Design review of the part built by this model. Coordinates are the model's own, in mm. A direction names the side the tool comes from. Give positions to 0.01 mm unless a question says otherwise; leave off trailing zeros. Write each loop counter-clockwise with the first axis right and the second up, starting at its lowest first coordinate (ties: lowest second). Pieces come first, ordered by that corner, then holes. Notation, with made-up numbers: (2, 74.5) -> (36, 74.5) arc R5 ccw to (36, 78.5) -> close; hole circle Ø8 at (37.5, 26.25). An arc over 180 degrees is marked (long way). Use CSV: the item, a comma, the result in double quotes.
```python
from build123d import *

# Parameters (mm, degrees)
SKETCH1_R           = 2.725
BOSS_EXTRUDE1_DEPTH = 2.9
SKETCH2_R           = 1.475
BOSS_EXTRUDE2_DEPTH = 10
CUT_EXTRUDE1_DEPTH  = 1.75


with BuildPart() as part:
    # Sketch1 → Boss-Extrude1 (new body)
    with BuildSketch(Plane(origin=(0, 0, 0), x_dir=(1, 0, 0), z_dir=(0, 1, 0))):
        Circle(SKETCH1_R)
    extrude(amount=BOSS_EXTRUDE1_DEPTH)

    # Sketch2 → Boss-Extrude2 (add)
    with BuildSketch(Plane.XZ):
        Circle(SKETCH2_R)
    extrude(amount=BOSS_EXTRUDE2_DEPTH)

    # Sketch3 → Cut-Extrude1 (cut)
    with BuildSketch(Plane(origin=(0, 2.9, 0), x_dir=(1, 0, 0), z_dir=(0, 1, 0))):
        Polygon((0, 1.443375673), (-1.25, 0.721687836), (-1.25, -0.721687836), (0, -1.443375673), (1.25, -0.721687836), (1.25, 0.721687836), align=None)
    extrude(amount=-CUT_EXTRUDE1_DEPTH, mode=Mode.SUBTRACT)


solid = part.part
```
(1) Take a section at C-C (x = 0.95). Write out the cut boundary in (y, z), then the cut area to 3 significant figures.
Established:
outline,"(-10, -1.13) -> (0, -1.13) -> (0, -2.55) -> (2.9, -2.55) -> (2.9, -0.89) -> (1.15, -0.89) -> (1.15, 0.89) -> (2.9, 0.89) -> (2.9, 2.55) -> (0, 2.55) -> (0, 1.13) -> (-10, 1.13) -> close"
area,"34.2 mm2"
(2) Tool access review of faces 1 (the face through (-1.474, -4.93, 0.065)), 2 (the face through (-0.64, 2.9, -1.25)), 3 (the face through (0.63, 2.04, -1.08)): name each direction out of +Z, -Z, +X, -X, +Y, -Y from which nothing blocks a thin tool from reaching the whole face with its end or side.
Established:
face 1,"-Y"
face 2,"+Z, -Z, +X, -X, +Y"
face 3,"+Y"
(3) Mouldability with a two-part tool opening along Z and no side actions: class faces 4 (the face through (0.616, 2.037, 1.088)), 5 (the face through (-1.25, 2, 0)), 6 (the face through (2.6, 1.43, -0.82)), 7 (the face through (0, -10, 0)) as +Z half, -Z half, draft (parallel to the pull), parting line (faces both ways), or undercut.
Established:
face 4,"undercut"
face 5,"undercut"
face 6,"parting line"
face 7,"draft"
(4) Take a section at A-A (z = 0). Write out the cut boundary in (x, y) (3 decimals).
Established:
outline,"(-2.725, 0) -> (-1.475, 0) -> (-1.475, -10) -> (1.475, -10) -> (1.475, 0) -> (2.725, 0) -> (2.725, 2.9) -> (1.25, 2.9) -> (1.25, 1.15) -> (-1.25, 1.15) -> (-1.25, 2.9) -> (-2.725, 2.9) -> close"
(5) For line 1 along Y through (x, z) = (0.25, -2.1); line 2 along Z through (x, y) = (-0.4, 1.5); line 3 along Z through (x, y) = (-0.1, -1.5), list the stretches that pass through material, from the lowest coordinate up. Write a range as [from, to].
Established:
line 1,"y = [0, 2.9]"
line 2,"z = [-2.7, -1.21], [1.21, 2.7]"
line 3,"z = [-1.47, 1.47]"
(6) Take a section at B-B (y = 0.5). Write out the cut boundary in (x, z) (3 decimals).
Established:
outline,"circle Ø5.45 at (0, 0)"
(7) Take a section at D-D (y = -2). Write out the cut boundary in (x, z) (3 decimals), then the cut area to 3 significant figures.
Established:
outline,"circle Ø2.95 at (0, 0)"
area,"6.83 mm2"
(8) Clearance check with flat-ended pins moving along their axes: pin 1 (2 mm diameter, centred on y = -5, z = -0.5, fed in from +X) (3 decimals); pin 2 (2 mm diameter, centred on x = 1.5, y = -7.5, fed in from +Z). State where each tip first meets the part, or that it passes through.
Established:
pin 1,"stops at x = 1.475"
pin 2,"stops at z = 1.39"
